Build history of the part. All positions in model axes, mm. A direction names the side the tool comes from. Coordinates: 2 decimals unless noted, no trailing zeros. Order: outer loops, then holes, each group sorted by start corner. A loop starts at its lowest first (then second) coordinate and runs counter-clockwise, first axis right, second up. Notation, with made-up numbers: (52, -28.75) - (88, -28.75) arc R24 ccw to (88, -8.75) - close; hole circle Ø9 at (42, -20.75). An arc over 180 degrees is marked (long way). Write each question's results on one line, items separated by ' | '.
from build123d import *

# Parameters (mm, degrees)
F0_W          = 66.1686062813
F0_H          = 70.2235847712
F1_DEPTH      = 25.4
F2_DEPTH      = 30.734
F2_DEPTH_BACK = 6.604
F0_W_2        = 7.764685899
F0_H_2        = 9.111225605
F3_DEPTH      = 33.274
F3_DEPTH_BACK = 7.62
F0_W_3        = 13.5037973523
F0_H_3        = 8.7774693966
F4_DEPTH      = 39.116
F4_DEPTH_BACK = 17.272


with BuildPart() as f1:
    # F0 (on Front) → F1 (new body)
    with BuildSketch(Plane.XZ):
        with BuildLine():
            ThreePointArc((33.0843031406, 44.2230179906), (0, 77.3073211312), (-33.0843031406, 44.2230179906))
            Line((-33.0843031406, 44.2230179906), (33.0843031406, 44.2230179906))
        make_face()
        with Locations((0, 9.111225605)):
            Rectangle(F0_W, F0_H)
    extrude(amount=F1_DEPTH)

    # F0 (on Front) → F2 (join, two sides)
    with BuildSketch(Plane.XZ) as f2_sk:
        with BuildLine():
            Line((-39.7869050503, 44.2230179906), (-33.0843031406, 44.2230179906))
            ThreePointArc((-33.0843031406, 44.2230179906), (0, 77.3073211312), (33.0843031406, 44.2230179906))
            Line((33.0843031406, 44.2230179906), (39.7869050503, 44.2230179906))
            ThreePointArc((39.7869050503, 44.2230179906), (0, 84.0099230409), (-39.7869050503, 44.2230179906))
        make_face()
    extrude(amount=F2_DEPTH)
    extrude(f2_sk.sketch, amount=-F2_DEPTH_BACK)

    # F0 (on Front) → F3 (join, two sides)
    with BuildSketch(Plane.XZ) as f3_sk:
        with Locations((36.9666460901, -30.5561795831)):
            Rectangle(F0_W_2, F0_H_2)
        with Locations((0, -30.5561795831)):
            Rectangle(F0_W, F0_H_2)
        with Locations((-36.9666460901, -30.5561795831)):
            Rectangle(F0_W_2, F0_H_2)
    extrude(amount=F3_DEPTH)
    extrude(f3_sk.sketch, amount=-F3_DEPTH_BACK)

    # F0 (on Front) → F4 (join, two sides)
    with BuildSketch(Plane.XZ) as f4_sk:
        with Locations((47.6008877158, -39.5005270839)):
            Rectangle(F0_W_3, F0_H_3)
        with Locations((36.9666460901, -39.5005270839)):
            Rectangle(F0_W_2, F0_H_3)
        with Locations((0, -39.5005270839)):
            Rectangle(F0_W, F0_H_3)
        with Locations((-36.9666460901, -39.5005270839)):
            Rectangle(F0_W_2, F0_H_3)
        with Locations((-47.6008877158, -39.5005270839)):
            Rectangle(F0_W_3, F0_H_3)
    extrude(amount=F4_DEPTH)
    extrude(f4_sk.sketch, amount=-F4_DEPTH_BACK)


solid = f1.part
1. Probe line 1 (Y direction, x = 7, z = -9); line 2 (Y direction, x = -13, z = -29.5); line 3 (X direction, y = -2, z = 1). List the from-to ranges inside material, lowest first.
Solved:
line 1: y = -25.4 to 0 | line 2: y = -33.27 to 7.62 | line 3: x = -33.08 to 33.08
2. Drop flat-ended pins along their axis: pin 1 Ø2.5 at (x, z) = (18, -31) entering from -Y; pin 2 Ø12 at (x, z) = (-29.5, -2) entering from +Y; pin 3 Ø12 at (x, y) = (30, -9.5) entering from +Z. Give the stop position or say it passes through.
Solved:
pin 1: stops at y = -33.27 | pin 2: stops at y = 0 | pin 3: stops at z = 75.96
3. Band-saw the part on C-C on x = 0. Give the cut face in (y, z), then the cut area to 3 significant figures.
Solved:
outline: (-39.12, -43.89) - (17.27, -43.89) - (17.27, -35.11) - (7.62, -35.11) - (7.62, -26) - (0, -26) - (0, 77.31) - (6.6, 77.31) - (6.6, 84.01) - (-30.73, 84.01) - (-30.73, 77.31) - (-25.4, 77.31) - (-25.4, -26) - (-33.27, -26) - (-33.27, -35.11) - (-39.12, -35.11) - close | area: 3,740 mm2
4. Tool access for faces 1 (the face through (33.084, -13, 9)), 2 (the face through (-1, 7.62, -30)), 3 (the face through (-36, -12, 44.223)), 4 (the face through (-3.1, -30.734, 77.5)): list every direction of +Z, -Z, +X, -X, +Y, -Y with a clear straight run to the whole face (end or side of a thin tool).
Solved:
face 1: +X, +Y, -Y | face 2: +Z, +X, -X, +Y | face 3: -X, +Y, -Y | face 4: +Z, +X, -X, -Y
5. Band-saw the part on D-D on z = 62. Give the cut face in (x, y).
Solved:
outline: (-35.59, -30.73) - (-27.9, -30.73) - (-27.9, -25.4) - (27.9, -25.4) - (27.9, -30.73) - (35.59, -30.73) - (35.59, 6.6) - (27.9, 6.6) - (27.9, 0) - (-27.9, 0) - (-27.9, 6.6) - (-35.59, 6.6) - close
6. Two-plate mould, pull along X, no slides. Class faces 5 (the face through (-1, -33.274, -30)), 6 (the face through (54.353, -11, -40)), 7 (the face through (0, 0, 26)): +X half, -X half, draft (parallel to the pull), parting line (faces both ways), or undercut.
Solved:
face 5: draft | face 6: +X half | face 7: undercut
7. Band-saw the part on A-A on y = 3. Give the cut face in (x, z).
Solved:
outline: (-54.35, -43.89) - (54.35, -43.89) - (54.35, -35.11) - (40.85, -35.11) - (40.85, -26) - (-40.85, -26) - (-40.85, -35.11) - (-54.35, -35.11) - close; (-39.79, 44.22) - (-33.08, 44.22) arc R33.08 cw to (33.08, 44.22) - (39.79, 44.22) arc R39.79 ccw to start
8. Band-saw the part on B-B on y = -10. Give the cut face in (x, z).
Solved:
outline: (-54.35, -43.89) - (54.35, -43.89) - (54.35, -35.11) - (40.85, -35.11) - (40.85, -26) - (33.08, -26) - (33.08, 44.22) - (39.79, 44.22) arc R39.79 ccw to (-39.79, 44.22) - (-33.08, 44.22) - (-33.08, -26) - (-40.85, -26) - (-40.85, -35.11) - (-54.35, -35.11) - close
